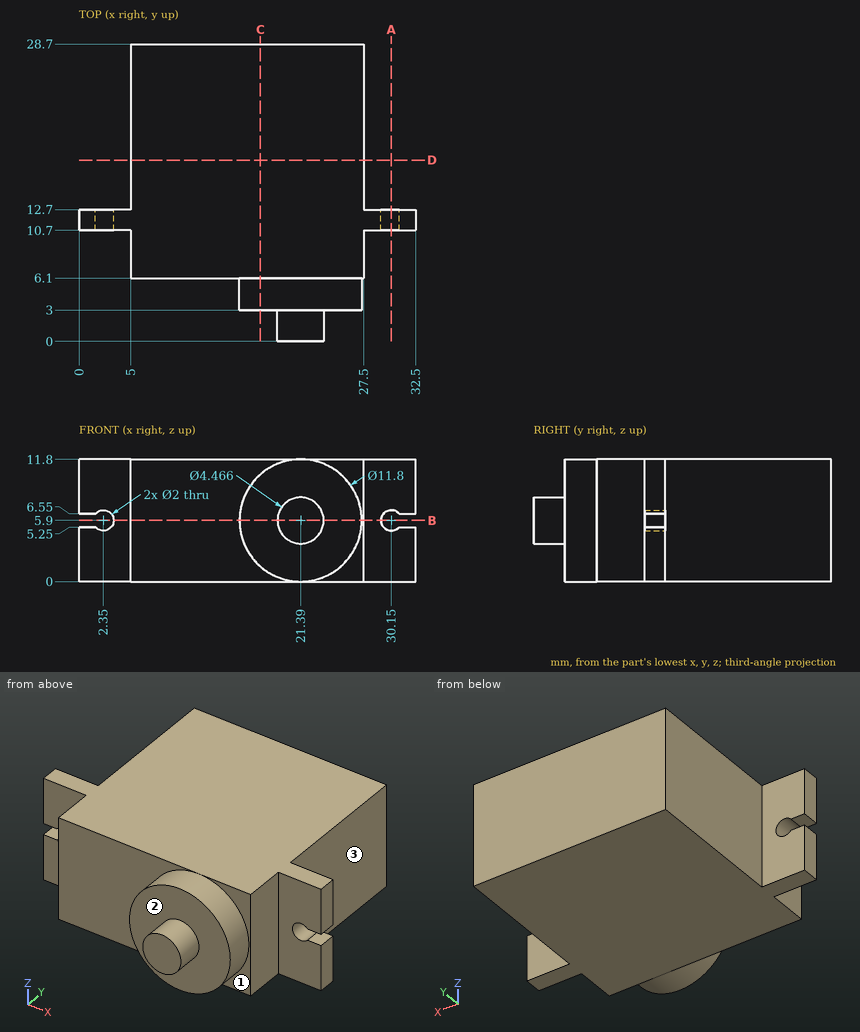
Source: three-view drawing plus pictorial views. Frame: mm from the lowest corner of the part. A direction names the side the tool comes from. Round coordinates to 2 decimals unless told otherwise and drop trailing zeros. Order: outer loops, then holes, each group sorted by start corner. A loop starts at its lowest first (then second) coordinate and runs counter-clockwise, first axis right, second up. Notation, with made-up numbers: M -5,4.25 L 44,4.25 A13 ccw 44,21.25 Z; hole C -26.75,67 d3. An arc over 180 degrees is marked long. One line per item, written item: value.
(1) Pin query (flat end, axial travel): P1, Ø1.5, axis at x = 10.5, z = 3.5, coming from the -Y side; P2, Ø1.5, axis at x = 3.5, z = 7, coming from the -Y side; P3, Ø5, axis at y = 7.5, z = 6.5, coming from the -X side; P4, Ø1.2, axis at x = 30.15, z = 5.9, coming from the +Y side. Return the tip coordinate at first contact, or that it passes through.
Result sheet:
P1: y = 6.1
P2: y = 10.7
P3: x = 5
P4: through
(2) Line query: probe 1 along Z at (x, y) = (2.35, 11.6); probe 2 along Y at (x, z) = (1, 3.5); probe 3 along Y at (x, z) = (10.5, 1.5). Output: solid intervals per line, ascending. Write a range as [from, to].
Result sheet:
probe 1: [0, 4.9], [6.9, 11.8]
probe 2: [10.7, 12.7]
probe 3: [6.1, 28.7]
(3) Cut plane D-D (y = 17.5). Return the cut outline in (x, z).
Result sheet:
outline: M 5,0 L 27.5,0 L 27.5,11.8 L 5,11.8 Z
(4) Reachability of the marked faces 1, 2 and 3 from +Z, -Z, +X, -X, +Y, -Y: full face, straight path, thin tool, end or side. Return the list, or none.
Result sheet:
face 1: +X, -Y
face 2: -Y
face 3: +Z, -Z, +X, +Y
(5) Cut plane B-B (z = 5.9). Return the cut outline in (x, y).
Result sheet:
outline: M 3.35,10.7 L 5,10.7 L 5,6.1 L 15.49,6.1 L 15.49,3 L 19.16,3 L 19.16,0 L 23.62,0 L 23.62,3 L 27.29,3 L 27.29,6.1 L 27.5,6.1 L 27.5,10.7 L 29.15,10.7 L 29.15,12.7 L 27.5,12.7 L 27.5,28.7 L 5,28.7 L 5,12.7 L 3.35,12.7 Z
(6) Cut plane A-A (x = 30.15). Return the cut outline in (y, z), and give its area (3 significant figures).
Result sheet:
outline: M 10.7,0 L 12.7,0 L 12.7,4.9 L 10.7,4.9 Z; M 10.7,6.9 L 12.7,6.9 L 12.7,11.8 L 10.7,11.8 Z
area: 19.6 mm2
(7) Cut plane C-C (x = 17.5). Return the cut outline in (y, z) (1 decimal), and give its area (3 significant figures).
Result sheet:
outline: M 3,1.5 L 6.1,1.5 L 6.1,0 L 28.7,0 L 28.7,11.8 L 6.1,11.8 L 6.1,10.3 L 3,10.3 Z
area: 294 mm2
